Build history of the part. All positions in model axes, mm. A direction names the side the tool comes from. Coordinates: 2 decimals unless noted, no trailing zeros. Write each loop counter-clockwise with the first axis right and the second up, starting at its lowest first coordinate (ties: lowest second). Pieces come first, ordered by that corner, then holes.
```python
from build123d import *

# Parameters (mm, degrees)
F1_DEPTH = 3
F2_W     = 1.4
F2_H     = 1.4
F3_DEPTH = 1.2
F4_R     = 0.5
F5_W     = 0.8
F5_H     = 1
F6_DEPTH = 8
F7_W     = 0.5999999121
F7_H     = 0.5
F8_DEPTH = 3
F9_R     = 0.2


with BuildPart() as f1:
    # F0 (on Top) → F1 (new body)
    with BuildSketch(Plane.XY):
        Polygon((0, 0.8), (0, 0), (8, 0), (8, 0.8), (5.5, 0.8), (5.5, 2), (2.5, 2), (2.5, 0.8), align=None)
    extrude(amount=F1_DEPTH)

    # F2 (on face) → F3 (cut)
    with BuildSketch(Plane.XZ):
        with Locations((4, 1.5)):
            Rectangle(F2_W, F2_H)
    extrude(amount=-F3_DEPTH, mode=Mode.SUBTRACT)

    # F4
    f4_edges = [f1.edges().sort_by_distance(p)[0] for p in [
        (5.5, 1.4, 3),
        (2.5, 1.4, 3),
        (2.5, 1.4, 0),
        (5.5, 1.4, 0),
    ]]
    fillet(f4_edges, radius=F4_R)

    # F5 (on face) → F6 (join, through all)
    with BuildSketch(Plane.YZ.offset(8)):
        with Locations((0.4, 3.5)):
            Rectangle(F5_W, F5_H)
    extrude(amount=-F6_DEPTH)

    # F7 (on face) → F8 (cut, through all)
    with BuildSketch(Plane.XY.offset(3)):
        with Locations((4, 1.75)):
            Rectangle(F7_W, F7_H)
    extrude(amount=-F8_DEPTH, mode=Mode.SUBTRACT)

    # F9
    f9_edges = [f1.edges().sort_by_distance(p)[0] for p in [
        (3.35, 2, 3),
        (4.65, 2, 3),
        (5.353553, 2, 2.853553),
        (5.5, 2, 1.5),
        (5.353553, 2, 0.146447),
        (3.35, 2, 0),
        (4.65, 2, 0),
        (2.646447, 2, 0.146447),
        (2.5, 2, 1.5),
        (2.646447, 2, 2.853553),
    ]]
    fillet(f9_edges, radius=F9_R)


solid = f1.part
```
1. Saw through at C-C on x = 4. List the corners of the cut face in (y, z).
Computed values:
outline: (0, 0) - (1.5, 0) - (1.5, 3) - (0.8, 3) - (0.8, 4) - (0, 4) - (0, 2.2) - (1.2, 2.2) - (1.2, 0.8) - (0, 0.8) - close
2. Saw through at D-D on y = 0.6. List the corners of the cut face in (x, z).
Computed values:
outline: (0, 0) - (8, 0) - (8, 4) - (0, 4) - close; hole (3.3, 0.8) - (4.7, 0.8) - (4.7, 2.2) - (3.3, 2.2) - close
3. Mould opens along X. For faces 1 (the face through (4, 1, 0.8)), 2 (the face through (5.5, 1, 1)), 3 (the face through (3, 2, 1)) say: +X half, -X half, draft (parallel to the pull), parting line (faces both ways), or undercut.
Computed values:
face 1: undercut
face 2: +X half
face 3: draft
4. Saw through at B-B on z = 1.6. List the corners of the cut face in (x, y).
Computed values:
outline: (0, 0) - (3.3, 0) - (3.3, 1.2) - (4.7, 1.2) - (4.7, 0) - (8, 0) - (8, 0.8) - (5.5, 0.8) - (5.5, 1.8) arc R0.2 ccw to (5.3, 2) - (4.3, 2) - (4.3, 1.5) - (3.7, 1.5) - (3.7, 2) - (2.7, 2) arc R0.2 ccw to (2.5, 1.8) - (2.5, 0.8) - (0, 0.8) - close
5. Saw through at A-A on y = 1.1. List the corners of the cut face in (x, z), plus the area to 3 significant figures.
Computed values:
outline: (2.5, 0.5) arc R0.5 ccw to (3, 0) - (5, 0) arc R0.5 ccw to (5.5, 0.5) - (5.5, 2.5) arc R0.5 ccw to (5, 3) - (3, 3) arc R0.5 ccw to (2.5, 2.5) - close; hole (3.3, 0.8) - (4.7, 0.8) - (4.7, 2.2) - (3.3, 2.2) - close
area: 6.83 mm2
6. Flat gauge pins, fed straight in: pin 1 (0.6 mm diameter, centred on y = 1.5, z = 1, fed in from -X); pin 2 (1.1 mm diameter, centred on x = 4.5, y = 1.5, fed in from +Z); pin 3 (0.5 mm diameter, centred on x = 4, z = 1.5, fed in from +Y). Where does each tip first touch, or does it go through?
Computed values:
pin 1: stops at x = 2.5
pin 2: stops at z = 3
pin 3: stops at y = 1.5
7. 3-axis set-ups, long thin cutter, end or side, ignore diameter. For faces 4 (the face through (4, 1, 3)), 5 (the face through (2.5, 1, 1)), 6 (the face through (4.7, 1, 1)): which of +Z, -Z, +X, -X, +Y, -Y reach the whole face in a straight line?
Computed values:
face 4: +Z, +X, -X, +Y
face 5: +Z, -Z, -X, +Y
face 6: -Y
8. Probe line 1 along Z through (x, y) = (4.5, 0.2); line 2 along X through (y, z) = (0.5, 1.1); line 3 along X through (y, z) = (1.7, 0.55). List the from-to ranges inside material, lowest first.
Computed values:
line 1: z = 0 to 0.8, 2.2 to 4
line 2: x = 0 to 3.3, 4.7 to 8
line 3: x = 2.5 to 3.7, 4.3 to 5.5
